Here's how the part is built. I have some questions about the finished solid (model axes, mm). A direction names the side the tool comes from. Give positions to 0.01 mm unless a question says otherwise; leave off trailing zeros. Loops run counter-clockwise (first coordinate to the right, second up) from the corner with the lowest first, then second, coordinate; pieces in that order, holes last.
Q1. I'm going to push flat-ended pins straight in: P1, Ø3, axis at x = 0, z = 0, coming from the -Y side; P2, Ø3, axis at x = 14.5, z = 0.5, coming from the +Y side; P3, Ø3, axis at y = 16.5, z = -5.5, coming from the +X side. Where does each tip first touch, or does it pass through?
Q2. For faces 5 (the face through (-3, 5, 8)), 6 (the face through (-6, -9, 0)), 7 (the face through (35, 40, 0)), which set-ups out of +Z, -Z, +X, -X, +Y, -Y let a thin tool reach every point of the face, with its end or its side?
Q3. Thinking about a two-plate mould opening in X: for faces 1 (the face through (-3, 5, -8)), 2 (the face through (-6.44, 0.52, 3.67)), 3 (the face through (-38.11, 49.03, 0.11)), 4 (the face through (31.66, 39.4, -0.11)), which applies, pulls with the +X half, pulls with the -X half, needs draft (parallel to the pull), parting line crosses it, or undercut?
Q4. I need wall thicknesses on probe 1 along Z at (x, y) = (0, -11); probe 2 along X at (y, z) = (-4.25, 0); probe 3 along X at (y, z) = (38, 4.5). Which ranges of each line are inside material? Lowest first, please.
Q5. Suppose I cut it at A-A (z = 0). List the corners of the cut face in (x, y) for me, and give its area (3 significant figures).
```python
from build123d import *

# Parameters (mm, degrees)
PAD_DEPTH     = 8
SKETCH002_R   = 7
PAD001_DEPTH  = 4.5
POCKET_DEPTH  = 5
SKETCH005_R   = 6
SKETCH005_R_2 = 2.6
PAD002_DEPTH  = 10
FILLET_R      = 4


with BuildPart() as part:
    # Sketch001 → Pad (new body, symmetric)
    with BuildSketch(Plane.XY):
        with BuildLine():
            ThreePointArc((-28.284271, 50), (-5.073059, 10.432043), (30, 40))
            Line((30, 40), (40, 40))
            ThreePointArc((-38.729833, 50), (-5.040172, 0.318812), (40, 40))
            Line((-38.729833, 50), (-28.284271, 50))
        make_face()
    extrude(amount=PAD_DEPTH, both=True)

    # Sketch002 → Pad001 (join, symmetric)
    with BuildSketch(Plane.XZ):
        Circle(SKETCH002_R)
    extrude(amount=PAD001_DEPTH, both=True)

    # Sketch004 (on Face8 of Pad001) → Pocket (cut)
    with BuildSketch(Plane.XZ.offset(4.5)):
        with BuildLine():
            Line((-1.532971, 2.1), (1.532971, 2.1))
            ThreePointArc((1.532971, -2.1), (2.6, 0), (1.532971, 2.1))
            Line((-1.532971, -2.1), (1.532971, -2.1))
            ThreePointArc((-1.532971, 2.1), (-2.6, 0), (-1.532971, -2.1))
        make_face()
    extrude(amount=-POCKET_DEPTH, mode=Mode.SUBTRACT)

    # Sketch005 (on Face8 of Pocket) → Pad002 (join)
    with BuildSketch(Plane.XZ.offset(4.5)):
        Circle(SKETCH005_R)
        Circle(SKETCH005_R_2, mode=Mode.SUBTRACT)
    extrude(amount=PAD002_DEPTH)

    # Fillet
    fillet_edges = [part.edges().sort_by_distance(p)[0] for p in [
        (-28.284271, 50, 0),
        (30, 40, 0),
        (-5.073059, 10.432043, -8),
        (-5.073059, 10.432043, 8),
        (-38.729833, 50, 0),
        (40, 40, 0),
    ]]
    fillet(fillet_edges, radius=FILLET_R)


solid = part.part
```
Solutions:
1. P1: stops at y = 0.5
1. P2: stops at y = 14.62
1. P3: stops at x = 33.41
2. face 5: +Z, +X, -X, +Y, -Y
2. face 6: -Y
2. face 7: +Z, -Z, +X, +Y
3. face 1: needs draft
3. face 2: parting line crosses it
3. face 3: pulls with the -X half
3. face 4: undercut
4. probe 1: z = -6 to -2.6, 2.6 to 6
4. probe 2: x = -7 to -2.6, 2.6 to 7
4. probe 3: x = -39.95 to -29.96, 30.3 to 39.24
5. outline: (-39.44, 46.67) arc R40 ccw to (-7, 0.62) - (-7, -4.5) - (-6, -4.5) - (-6, -14.5) - (-2.6, -14.5) - (-2.6, 0.5) - (2.6, 0.5) - (2.6, -14.5) - (6, -14.5) - (6, -4.5) - (7, -4.5) - (7, 0.62) arc R40 ccw to (39.75, 35.56) arc R4 ccw to (35.78, 40) - (33.76, 40) arc R4 ccw to (29.79, 36.47) arc R30 cw (long way) to (-29.53, 45.29) arc R4 ccw to (-33.47, 50) - (-35.5, 50) arc R4 ccw to start
5. area: 1,290 mm2
